CAD build for the part. Positions are in the model's coordinates, mm. A direction names the side the tool comes from. Coordinates: 2 decimals unless noted, no trailing zeros. Order: outer loops, then holes, each group sorted by start corner. A loop starts at its lowest first (then second) coordinate and runs counter-clockwise, first axis right, second up. Notation, with made-up numbers: (63.5, 57.5) - (82.5, 57.5) arc R15 cw to (82.5, 80.5) - close; hole circle Ø11 at (17.5, 13.25). An arc over 180 degrees is marked (long way). Write each question's results on one line, items separated by ' | '. Start each with the question number.
Q1. Wall check: probe 1 along Z at (x, y) = (9, -5); probe 2 along Y at (x, z) = (6, 13.5); probe 3 along Y at (x, z) = (4, 14). Give the ranges that are in metal, low to high.
Q2. Band-saw the part on B-B, the plane z = 3. Write the cut outline in (x, y), then the cut area to 3 significant figures.
Q3. Pin check, flat tips, straight feed: P1, Ø12, axis at x = -20, y = -20, coming from the +Z side; P2, Ø8.5, axis at x = -12, y = -22, coming from the -Z side; P3, Ø9.5, axis at x = -2, z = -5.5, coming from the -Y side. Stop position of each tip, or through.
Q4. Band-saw the part on C-C, the plane y = -24.5. Write the cut outline in (x, z), then the cut area to 3 significant figures.
Q5. Which spindle directions (+Z, -Z, +X, -X, +Y, -Y) get a long thin tool onto all of the face, cutting with end or side? Do faces 1 (the flat face through (0, -3.5, 8)), 2 (the flat face through (-25, -10, 0)), 3 (the flat face through (0, -17, -1.75)). Say none if no direction does.
Q6. Band-saw the part on A-A, the plane x = 1. Write the cut outline in (y, z), then the cut area to 3 significant figures.
```python
from build123d import *

# Parameters (mm, degrees)
F0_W        = 50
F0_H        = 30
F1_DEPTH    = 3.5
F2_R        = 1.5
F3_W        = 50
F3_H        = 3.5
F4_DEPTH    = 30
F5_T1_DEPTH = 60


# Not quite as in the source:
# - a fillet or chamfer that OpenCascade refuses, or shapes differently, is made with other operations: its cross-section is extruded or revolved along the edge and cut away or added


with BuildPart() as f1:
    # F0 (on Front) → F1 (new body)
    with BuildSketch(Plane.XZ):
        Rectangle(F0_W, F0_H)
    extrude(amount=F1_DEPTH)

    # F2
    f2_edges = [f1.edges().sort_by_distance(p)[0] for p in [
        (0, -3.5, 15),
        (0, -3.5, -15),
    ]]
    fillet(f2_edges, radius=F2_R)

    # F3 (on face) → F4 (join)
    with BuildSketch(Plane.XZ.offset(3.5)):
        Rectangle(F3_W, F3_H)
    extrude(amount=F4_DEPTH)

    # F5: fillet of radius 2 on 2 edges, made by hand

    # F5_s2 → F5_t1 (cut)
    with BuildSketch(Plane.YZ.offset(-30)):
        with BuildLine():
            ThreePointArc((-31.5, -1.75), (-32.9142135624, -1.1642135624), (-33.5, 0.25))
            Line((-33.5, 0.25), (-33.5, -1.75))
            Line((-33.5, -1.75), (-31.5, -1.75))
        make_face()
        with BuildLine():
            ThreePointArc((-31.5, 1.75), (-32.9142135624, 1.1642135624), (-33.5, -0.25))
            Line((-33.5, -0.25), (-33.5, 1.75))
            Line((-33.5, 1.75), (-31.5, 1.75))
        make_face()
    extrude(amount=F5_T1_DEPTH, mode=Mode.SUBTRACT)


solid = f1.part
```
Results below:
1) probe 1: z = -1.75 to 1.75 | probe 2: y = -3.5 to 0 | probe 3: y = -3.41 to 0
2) outline: (-25, -3.5) - (25, -3.5) - (25, 0) - (-25, 0) - close | area: 175 mm²
3) P1: stops at z = 1.75 | P2: stops at z = -1.75 | P3: stops at y = -33.23
4) outline: (-25, -1.75) - (25, -1.75) - (25, 1.75) - (-25, 1.75) - close | area: 175 mm²
5) face 1: +Z, +X, -X, -Y | face 2: +Z, -Z, -X, +Y, -Y | face 3: -Z, +X, -X, -Y
6) outline: (-33.48, 0) arc R2 ccw to (-31.5, -1.75) - (-3.5, -1.75) - (-3.5, -13.5) arc R1.5 ccw to (-2, -15) - (0, -15) - (0, 15) - (-2, 15) arc R1.5 ccw to (-3.5, 13.5) - (-3.5, 1.75) - (-31.5, 1.75) arc R2 ccw to start | area: 207 mm²
